Part model, mm, in its own coordinate system. A direction names the side the tool comes from. Coordinates: 2 decimals unless noted, no trailing zeros. Write each loop counter-clockwise with the first axis right and the second up, starting at its lowest first coordinate (ties: lowest second). Pieces come first, ordered by that corner, then holes. Notation, with made-up numbers: M -6,57 L 5,57 A28 ccw 5,75 Z; hole C 19.5,-12.75 d1. An arc over 180 degrees is marked long. Use a Markdown table: item, result. Add a question column.
Q1. Slice it at B-B on x = 0.5. Write the cut outline in (y, z), then the cut area to 3 significant figures.
Q2. Slice it at C-C on y = -162.5. Write the cut outline in (x, z).
Q3. Tool access for faces 1 (the flat face through (0, -75, -14)), 2 (the flat face through (0, -41, 6)): list every direction of +Z, -Z, +X, -X, +Y, -Y with a clear straight run to the whole face (end or side of a thin tool).
Q4. Pin check, flat tips, straight feed: pin 1 Ø1.5 at (x, y) = (2.5, -149.5) entering from +Z; pin 2 Ø4 at (x, z) = (0.5, 1.5) entering from -Y. Stop position of each tip, or through.
Q5. Wall check: L1, parallel to Y at x = -2.5, z = -7.5; L2, parallel to Y at x = 4, z = 2; L3, parallel to Z at x = 3, y = -140. Give the ranges that are in metal, low to high. Write a range as from..to.
Q6. Slice it at D-D on z = -4.25. Write the cut outline in (x, y), then the cut area to 3 significant figures.
Q7. Slice it at A-A on z = -17.25. Write the cut outline in (x, y).
Q8. Mould opens along Y. For faces 3 (the flat face through (0, -62, -14)), 4 (the flat face through (0, -138, -7)), 5 (the flat face through (0, -102, -1)), 6 (the flat face through (0, -68, -7)) say: released by +Y, released by -Y, zero draft, split by the parting line, or undercut.
from build123d import *

# Parameters (mm, degrees)
BOX039_W     = 13
BOX039_H     = 120
BOX039_DEPTH = 13
BOX038_W     = 13
BOX038_H     = 80
BOX038_DEPTH = 13
BOX040_W     = 13
BOX040_H     = 100
BOX040_DEPTH = 13


with BuildPart() as cube035:
    # Box039 → Box039 (new body)
    with BuildSketch(Plane(origin=(-6.5, -102, -7), x_dir=(1, 0, 0), z_dir=(0, 0, 1))):
        with Locations((6.5, 60)):
            Rectangle(BOX039_W, BOX039_H)
    extrude(amount=BOX039_DEPTH)


with BuildPart() as fusion020:
    # Box038 → Box038 (new body)
    with BuildSketch(Plane(origin=(-6.5, -62, -20), x_dir=(1, 0, 0), z_dir=(0, 0, 1))):
        with Locations((6.5, 40)):
            Rectangle(BOX038_W, BOX038_H)
    extrude(amount=BOX038_DEPTH)

    # Fusion020: union Cube035
    add(cube035.part)


with BuildPart() as fusion025:
    # Box040 → Box040 (new body)
    with BuildSketch(Plane(origin=(-6.5, -175, -20), x_dir=(1, 0, 0), z_dir=(0, 0, 1))):
        with Locations((6.5, 50)):
            Rectangle(BOX040_W, BOX040_H)
    extrude(amount=BOX040_DEPTH)

    # Fusion025: union Fusion020
    add(fusion020.part)


solid = fusion025.part
Recorded:
| question | item | result |
|---|---|---|
| 1 | outline | M -175,-20 L -75,-20 L -75,-7 L -62,-7 L -62,-20 L 18,-20 L 18,6 L -102,6 L -102,-7 L -175,-7 Z |
| 1 | area | 3,900 mm² |
| 2 | outline | M -6.5,-20 L 6.5,-20 L 6.5,-7 L -6.5,-7 Z |
| 3 | face 1 | -Z, +X, -X |
| 3 | face 2 | +Z, +X, -X, +Y, -Y |
| 4 | pin 1 | z = -7 |
| 4 | pin 2 | y = -102 |
| 5 | L1 | -175..-75, -62..18 |
| 5 | L2 | -102..18 |
| 5 | L3 | -20..-7 |
| 6 | outline | M -6.5,-102 L 6.5,-102 L 6.5,18 L -6.5,18 Z |
| 6 | area | 1,560 mm² |
| 7 | outline | M -6.5,-175 L 6.5,-175 L 6.5,-75 L -6.5,-75 Z; M -6.5,-62 L 6.5,-62 L 6.5,18 L -6.5,18 Z |
| 8 | face 3 | undercut |
| 8 | face 4 | zero draft |
| 8 | face 5 | released by -Y |
| 8 | face 6 | undercut |
